```python
from build123d import *

# Parameters (mm, degrees)
F1_DEPTH  = 5
F3_DEPTH  = 25
F5_R      = 2
F5_W      = 5.9894541353
F5_H      = 11.9529513837
F6_DEPTH  = 4
F8_DEPTH  = 10
F9_R      = 2
F10_DEPTH = 25


with BuildPart() as f1:
    # F0 (on Top) → F1 (new body)
    with BuildSketch(Plane.XY):
        with BuildLine():
            Line((0, 44), (0, 0))
            Line((0, 0), (26.4925560224, 0))
            Line((26.4925560224, 0), (32, 0))
            ThreePointArc((32, 0), (36, 4), (32, 8))
            Line((32, 8), (26.4925560224, 8))
            Line((26.4925560224, 8), (26.4925560224, 44))
            Line((26.4925560224, 44), (0, 44))
        make_face()
    extrude(amount=F1_DEPTH)

    # F2 (on face) → F3 (join)
    with BuildSketch(Plane(origin=(0, 8, 0), x_dir=(-1, 0, 0), z_dir=(0, 1, 0))):
        Polygon((-26.4925560224, 15), (-26.4925560224, 5), (-18.4925560224, 5), (-18.4925560224, 17.7138329376), (-2.2473606405, 35.1346721534), (12.0133898596, 35.1346721534), (12.0133898596, 39.1346721534), (-3.9866101404, 39.1346721534), align=None)
    extrude(amount=F3_DEPTH)

    # F5 (on offset) → F6 (join)
    with BuildSketch(Plane(origin=(21.6520220325, 0, 20.1908371907), x_dir=(0, 1, 0), z_dir=(0.7313537016, 0, 0.6819983601))):
        with BuildLine():
            Line((8, 14.9024257631), (4, 14.9024257631))
            ThreePointArc((4, 14.9024257631), (-2, 8.9024257631), (4, 2.9024257631))
            Line((4, 2.9024257631), (8, 2.9024257631))
            Line((8, 2.9024257631), (8, 2.9494743794))
            Line((8, 2.9494743794), (8, 14.9024257631))
        make_face()
        with Locations((4, 8.9024257631)):
            Circle(F5_R, mode=Mode.SUBTRACT)
        with Locations((10.9947270676, 8.9259500713)):
            Rectangle(F5_W, F5_H)
    extrude(amount=-F6_DEPTH)

    # F7 (on offset) → F8 (cut)
    with BuildSketch(Plane(origin=(21.6520220325, 0, 20.1908371907), x_dir=(0, 1, 0), z_dir=(0.7313537016, 0, 0.6819983601))):
        with BuildLine():
            ThreePointArc((30.2680338025, 16.9024257631), (29.2680338025, 17.9024257631), (28.2680338025, 16.9024257631))
            Line((28.2680338025, 16.9024257631), (28.2680338025, 2.9024257631))
            ThreePointArc((28.2680338025, 2.9024257631), (29.2680338025, 1.9024257631), (30.2680338025, 2.9024257631))
            Line((30.2680338025, 2.9024257631), (30.2680338025, 16.9024257631))
        make_face()
    extrude(amount=-F8_DEPTH, mode=Mode.SUBTRACT)

    # F9 (on Top) → F10 (cut)
    with BuildSketch(Plane.XY):
        with Locations((4.8117552102, 39.6364554763)):
            Circle(F9_R)
        with Locations((20.8117552102, 39.6364554763)):
            Circle(F9_R)
        with Locations((31.0607589781, 3.6364554763)):
            Circle(F9_R)
        with Locations((4.7061769292, 3.8695221301)):
            Circle(F9_R)
    extrude(amount=F10_DEPTH, mode=Mode.SUBTRACT)


solid = f1.part
```
For this review, take the finished solid that the model builds, in its own axes (mm). A direction names the side the tool comes from. Round coordinates to 2 decimals unless told otherwise and drop trailing zeros. Order: outer loops, then holes, each group sorted by start corner. A loop starts at its lowest first (then second) coordinate and runs counter-clockwise, first axis right, second up. Notation, with made-up numbers: (63.5, 70.25) -> (112.5, 70.25) arc R20 ccw to (112.5, 99.25) -> close; hole circle Ø3 at (24.25, 8.25). An arc over 180 degrees is marked (long way). Use a Markdown table: item, result.
Item 1: Take a section at B-B (x = 22). State the section outline as (y, z) points, plus the area to 3 significant figures.
Resolved:
| item | result |
|---|---|
| outline | (0, 0) -> (38.03, 0) -> (38.03, 5) -> (33, 5) -> (33, 19.82) -> (8, 19.82) -> (8, 5) -> (0, 5) -> close; (41.25, 0) -> (44, 0) -> (44, 5) -> (41.25, 5) -> close |
| area | 574 mm² |
Item 2: Draft analysis for pull direction X (two halves, no side actions). For faces 1 (the cylindrical face through (14.05, -2, 25.45)), 2 (the flat face through (-5, 20, 35.135)), 3 (the cylindrical face through (32.91, 2.87, 2.46)), state which applies: +X half, -X half, draft (parallel to the pull), parting line (faces both ways), or undercut.
Resolved:
| item | result |
|---|---|
| face 1 | parting line |
| face 2 | draft |
| face 3 | undercut |
Item 3: For line 1 along Z through (x, y) = (0.5, 20); line 2 along Y through (x, z) = (6, 4.5); line 3 along Y through (x, z) = (15.5, 25), list the stretches that pass through material, from the lowest coordinate up. Write a range as [from, to].
Resolved:
| item | result |
|---|---|
| line 1 | z = [0, 5], [35.13, 39.13] |
| line 2 | y = [0, 2.34], [5.39, 38.03], [41.25, 44] |
| line 3 | y = [-1.88, 2.39], [5.61, 28.27], [30.27, 33] |
Item 4: For pin 1 (3 mm diameter, centred on y = 24, z = 16.5, fed in from -X); pin 2 (10 mm diameter, centred on y = 22.5, z = 17.5, fed in from +X); pin 3 (7 mm diameter, centred on x = -8, y = 15.5, fed in from -Z); pin 4 (3.5 mm diameter, centred on x = 20.81, y = 39.64, fed in from -Z), all flat-tipped, find the tip position at first contact; note any pin that passes through.
Resolved:
| item | result |
|---|---|
| pin 1 | stops at x = 18.23 |
| pin 2 | stops at x = 26.49 |
| pin 3 | stops at z = 35.13 |
| pin 4 | passes through |
Item 5: Machinability: for faces 4 (the flat face through (26.493, 22, 8)), 5 (the flat face through (13, 33, 25)), 6 (the cylindrical face through (8, 29.29, 31.94)), 7 (the flat face through (16, 0, 2)), which of the approach directions +Z, -Z, +X, -X, +Y, -Y give a long, thin tool a straight path to every point of the face, cutting with its end or side? Answer none if there is none.
Resolved:
| item | result |
|---|---|
| face 4 | +Z, -Z, +X, +Y |
| face 5 | +Z, +X, -X, +Y |
| face 6 | +X |
| face 7 | -Z, +X, -X, -Y |
Item 6: Take a section at D-D (z = 4). State the section outline as (x, y) points.
Resolved:
| item | result |
|---|---|
| outline | (0, 0) -> (32, 0) arc R4 ccw to (32, 8) -> (26.49, 8) -> (26.49, 44) -> (0, 44) -> close; hole circle Ø4 at (4.71, 3.87); hole circle Ø4 at (4.81, 39.64); hole circle Ø4 at (20.81, 39.64); hole circle Ø4 at (31.06, 3.64) |
Item 7: Take a section at C-C (y = 1). State the section outline as (x, z) points.
Resolved:
| item | result |
|---|---|
| outline | (0, 0) -> (34.65, 0) -> (34.65, 5) -> (0, 5) -> close; (9.11, 27.77) -> (16.2, 20.17) -> (19.12, 22.9) -> (12.04, 30.5) -> close |
Item 8: Take a section at A-A (y = 11). State the section outline as (x, z) points.
Resolved:
| item | result |
|---|---|
| outline | (-12.01, 35.13) -> (2.25, 35.13) -> (18.49, 17.71) -> (18.49, 5) -> (0, 5) -> (0, 0) -> (26.49, 0) -> (26.49, 15) -> (3.99, 39.13) -> (-12.01, 39.13) -> close |
